Part model, mm, in its own coordinate system. Give positions to 0.01 mm unless a question says otherwise; leave off trailing zeros. Order: outer loops, then holes, each group sorted by start corner. A loop starts at its lowest first (then second) coordinate and runs counter-clockwise, first axis right, second up.
1. Mould opens along X. For faces 1 (the cylindrical face through (0.481, 7.418, 71.436)), 2 (the cylindrical face through (-1.73, -7.81, 59.16)), 3 (the flat face through (4, -6, 120)), 4 (the cylindrical face through (-1.42, -7.4, 15.74)) say: +X half, -X half, draft (parallel to the pull), parting line (faces both ways), or undercut.
2. Slice it at B-B on x = 0. List the corners of the cut face in (y, z).
3. Slice it at C-C on z = 69.91. List the corners of the cut face in (x, y).
4. Probe line 1 (Z direction, x = 0, y = 7.25); line 2 (Y direction, x = 0, z = 81); line 3 (Y direction, x = 2.5, z = 29). List the from-to ranges inside material, lowest first.
5. Slice it at D-D on z = 33. List the corners of the cut face in (x, y).
6. Slice it at A-A on y = 0. List the corners of the cut face in (x, z).
7. Drop flat-ended pins along their axis: pin 1 Ø3 at (x, y) = (0, -3.5) entering from -Z; pin 2 Ø5 at (x, z) = (0, 69.91) entering from -Y; pin 3 Ø1.5 at (y, z) = (4, 42) entering from +X; pin 4 Ø3 at (x, z) = (3, 56) entering from +Y. Give the stop position or say it passes through.
from build123d import *

# Parameters (mm, degrees)
SKETCH_1_R          = 8
SKETCH_1_R_2        = 7
EXTRUDE_1_DEPTH     = 120
SKETCH_2_R          = 1.6
CUT_EXTRUDE_1_DEPTH = 300


with BuildPart() as part:
    # 草图1 → 凸台-拉伸1 (new body)
    with BuildSketch(Plane.XY):
        Circle(SKETCH_1_R)
        Circle(SKETCH_1_R_2, mode=Mode.SUBTRACT)
    extrude(amount=EXTRUDE_1_DEPTH)

    # 草图2 → 切除-拉伸1 (cut, symmetric)
    with BuildSketch(Plane(origin=(0, 0, 0), x_dir=(1, 0, 0), z_dir=(0, 1, 0))):
        with Locations(Location((0, -15, 0), (0, 0, 270))):
            Circle(SKETCH_2_R)
        with Locations(Location((0, -69.91, 0), (0, 0, 270))):
            Circle(SKETCH_2_R)
    extrude(amount=CUT_EXTRUDE_1_DEPTH, both=True, mode=Mode.SUBTRACT)


solid = part.part
Data:
1. face 1: undercut
1. face 2: parting line
1. face 3: draft
1. face 4: undercut
2. outline: (-8, 0) - (-7, 0) - (-7, 13.4) - (-8, 13.4) - close; (-8, 16.6) - (-7, 16.6) - (-7, 68.31) - (-8, 68.31) - close; (-8, 71.51) - (-7, 71.51) - (-7, 120) - (-8, 120) - close; (7, 0) - (8, 0) - (8, 13.4) - (7, 13.4) - close; (7, 16.6) - (8, 16.6) - (8, 68.31) - (7, 68.31) - close; (7, 71.51) - (8, 71.51) - (8, 120) - (7, 120) - close
3. outline: (-1.6, -7.84) - (-1.6, -6.81) arc R7 cw to (-1.6, 6.81) - (-1.6, 7.84) arc R8 ccw to start; (1.6, -7.84) arc R8 ccw to (1.6, 7.84) - (1.6, 6.81) arc R7 cw to (1.6, -6.81) - close
4. line 1: z = 0 to 13.4, 16.6 to 68.31, 71.51 to 120
4. line 2: y = -8 to -7, 7 to 8
4. line 3: y = -7.6 to -6.54, 6.54 to 7.6
5. outline: circle Ø16 at (0, 0); hole circle Ø14 at (0, 0)
6. outline: (-8, 0) - (-7, 0) - (-7, 120) - (-8, 120) - close; (7, 0) - (8, 0) - (8, 120) - (7, 120) - close
7. pin 1: passes through
7. pin 2: stops at y = -8
7. pin 3: stops at x = 7.31
7. pin 4: stops at y = 7.86
